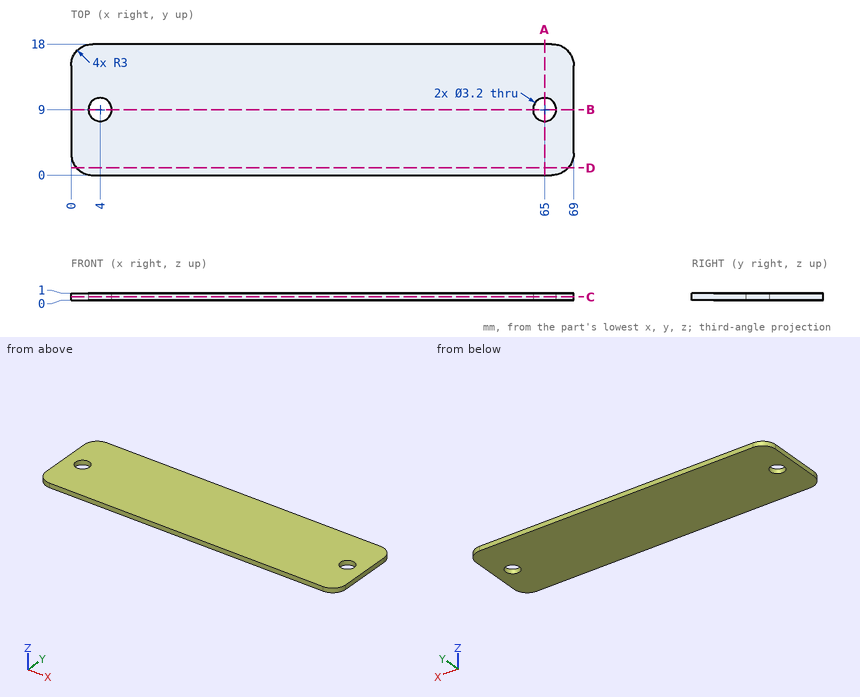
Geometry check sheet. Reference: drawing and pictorial views, mm from the part's lowest x, y, z. Coordinates: 2 decimals unless noted, no trailing zeros. Loops run counter-clockwise (first coordinate to the right, second up) from the corner with the lowest first, then second, coordinate; pieces in that order, holes last. Notation, with made-up numbers: (5, 75) -> (54, 75) arc R7 cw to (54, 86) -> close; hole circle Ø1 at (26.5, -12.75). An arc over 180 degrees is marked (long way). Put each result on its own line as item: value.
1) Cross-section at C-C on z = 0.5. Record the boundary of the cut face in (x, y).
Result set:
outline: (0, 3) arc R3 ccw to (3, 0) -> (66, 0) arc R3 ccw to (69, 3) -> (69, 15) arc R3 ccw to (66, 18) -> (3, 18) arc R3 ccw to (0, 15) -> close; hole circle Ø3.2 at (4, 9); hole circle Ø3.2 at (65, 9)
2) Thickness scan on line 1 (Y direction, x = 4, z = 0.4); line 2 (X direction, y = 7.75, z = 0.35); line 3 (X direction, y = 2.5, z = 0.7). Record the ranges inside material, lowest first.
Result set:
line 1: y = 0 to 7.4, 10.6 to 18
line 2: x = 0 to 3, 5 to 64, 66 to 69
line 3: x = 0.04 to 68.96
3) Cross-section at A-A on x = 65. Record the boundary of the cut face in (y, z).
Result set:
outline: (0, 0) -> (7.4, 0) -> (7.4, 1) -> (0, 1) -> close; (10.6, 0) -> (18, 0) -> (18, 1) -> (10.6, 1) -> close
4) Cross-section at B-B on y = 9. Record the boundary of the cut face in (x, z).
Result set:
outline: (0, 0) -> (2.4, 0) -> (2.4, 1) -> (0, 1) -> close; (5.6, 0) -> (63.4, 0) -> (63.4, 1) -> (5.6, 1) -> close; (66.6, 0) -> (69, 0) -> (69, 1) -> (66.6, 1) -> close
5) Gauge pin test, flat ends, axial feed: pin 1 Ø2 at (x, y) = (7, 6) entering from -Z; pin 2 Ø1.9 at (x, y) = (65, 9) entering from -Z. Record the tip position at first contact, or that the pin passes through.
Result set:
pin 1: stops at z = 0
pin 2: passes through
6) Cross-section at D-D on y = 1. Record the boundary of the cut face in (x, z).
Result set:
outline: (0.76, 0) -> (68.24, 0) -> (68.24, 1) -> (0.76, 1) -> close
